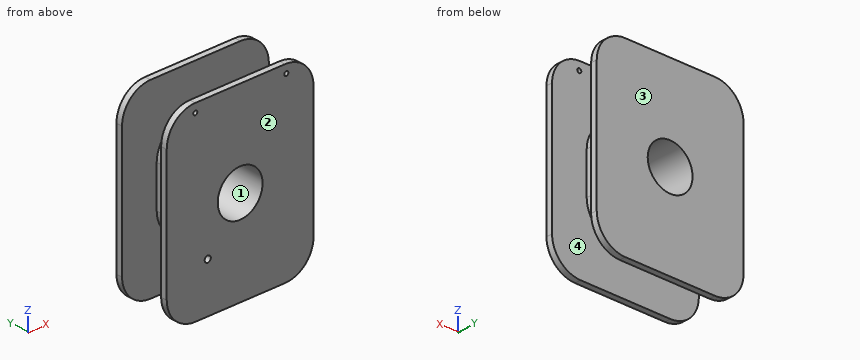
from build123d import *

# Parameters (mm, degrees)
F0_W      = 36
F0_H      = 45
F0_R      = 5.5
F1_DEPTH  = 1.5
F2_W      = 19
F2_H      = 24
F2_R      = 5.5
F3_DEPTH  = 12
F4_W      = 36
F4_H      = 45
F4_W_2    = 19
F4_H_2    = 24
F4_R      = 5.5
F5_DEPTH  = 1.5
F6_R      = 7
F7_R      = 0.75
F8_DEPTH  = 2.5
F9_R      = 0.5
F10_DEPTH = 2.5


# Not quite as in the source:
# - a feature names something its author has since deleted; it is built from what else it names


with BuildPart() as f1:
    # F0 (on Front) → F1 (new body)
    with BuildSketch(Plane.XZ):
        Rectangle(F0_W, F0_H)
        Circle(F0_R, mode=Mode.SUBTRACT)
    extrude(amount=F1_DEPTH)

    # F2 (on face) → F3 (join)
    with BuildSketch(Plane.XZ.offset(1.5)):
        Rectangle(F2_W, F2_H)
        Circle(F2_R, mode=Mode.SUBTRACT)
    extrude(amount=F3_DEPTH)

    # F4 (on face) → F5 (join)
    with BuildSketch(Plane.XZ.offset(13.5)):
        Rectangle(F4_W, F4_H)
        Rectangle(F4_W_2, F4_H_2, mode=Mode.SUBTRACT)
        Rectangle(F4_W_2, F4_H_2)
        Circle(F4_R, mode=Mode.SUBTRACT)
    extrude(amount=-F5_DEPTH)

    # F6
    f6_edges = [f1.edges().sort_by_distance(p)[0] for p in [
        (9.5, -6.75, 12),
        (9.5, -6.75, -12),
        (18, -0.75, 22.5),
        (18, -12.75, 22.5),
        (18, -12.75, -22.5),
        (18, -0.75, -22.5),
        (-18, -0.75, -22.5),
        (-18, -12.75, -22.5),
        (-9.5, -6.75, -12),
        (-9.5, -6.75, 12),
        (-18, -0.75, 22.5),
        (-18, -12.75, 22.5),
    ]]
    fillet(f6_edges, radius=F6_R)

    # F7 (on face) → F8 (cut)
    with BuildSketch(Plane.XZ.offset(13.5)):
        with Locations((-7.9445969313, -10.7102040201)):
            Circle(F7_R)
    extrude(amount=-F8_DEPTH, mode=Mode.SUBTRACT)

    # F9 (on face) → F10 (cut)
    with BuildSketch(Plane.XZ.offset(13.5)):
        with Locations((-11, 20.4497474683)):
            Circle(F9_R)
        with Locations((11.3213816658, 20.4497474683)):
            Circle(F9_R)
    extrude(amount=-F10_DEPTH, mode=Mode.SUBTRACT)


solid = f1.part
Can you work these out from the model? Positions are in its coordinate system, mm. Face numbers are marked on the shaded views. A direction names the side the tool comes from. Coordinates: 2 decimals unless noted, no trailing zeros. Write each loop counter-clockwise with the first axis right and the second up, starting at its lowest first coordinate (ties: lowest second). Pieces come first, ordered by that corner, then holes.
Q1. For P1, Ø0.9, axis at x = -7.94, z = -10.71, coming from the +Y side; P2, Ø5.5, axis at x = 1, y = -5, coming from the +Z side; P3, Ø2, axis at x = 3.5, y = -8.5, coming from the -Z side; P4, Ø3, axis at y = -7.5, z = 0, coming from the -X side, each with a flat end and sliding along its axis, tell me the tip position at first contact or that it passes through.
Results found:
P1: stops at y = 0
P2: stops at z = 12
P3: stops at z = -12
P4: stops at x = -9.5
Q2. Imagine slicing it at D-D, the plane z = 13. List the corners of the cut face in (x, y) for me, plus the area to 3 significant figures.
Results found:
outline: (-18, -13.5) - (18, -13.5) - (18, -12) - (-18, -12) - close; (-18, -1.5) - (18, -1.5) - (18, 0) - (-18, 0) - close
area: 108 mm2
Q3. Imagine slicing it at C-C, the plane x = 0. List the corners of the cut face in (y, z) for me.
Results found:
outline: (-13.5, -22.5) - (-12, -22.5) - (-12, -12) - (-1.5, -12) - (-1.5, -22.5) - (0, -22.5) - (0, -5.5) - (-13.5, -5.5) - close; (-13.5, 5.5) - (0, 5.5) - (0, 22.5) - (-1.5, 22.5) - (-1.5, 12) - (-12, 12) - (-12, 22.5) - (-13.5, 22.5) - close
Q4. Which directions (+Z, -Z, +X, -X, +Y, -Y) give clear straight access to the entire face, cutting with the end or side of a thin tool? Please do the marked faces 3 and 4.
Results found:
face 3: +Z, -Z, +X, -X, +Y
face 4: none
Q5. Imagine slicing it at B-B, the plane y = -7. List the corners of the cut face in (x, z) for me, plus the area to 3 significant figures.
Results found:
outline: (-9.5, -5) arc R7 ccw to (-2.5, -12) - (2.5, -12) arc R7 ccw to (9.5, -5) - (9.5, 5) arc R7 ccw to (2.5, 12) - (-2.5, 12) arc R7 ccw to (-9.5, 5) - close; hole circle Ø11 at (0, 0)
area: 319 mm2
Q6. Please list where these lines run through material, in increasing order: L1, parallel to Y at x = 15, z = 20.5; L2, parallel to Z at x = -11, y = -13.1; L3, parallel to Z at x = 0, y = -4.25.
Results found:
L1: y = -13.5 to -12, -1.5 to 0
L2: z = -22.5 to 19.95, 20.95 to 22.5
L3: z = -12 to -5.5, 5.5 to 12
Q7. If we mould it in two halves opening along X, with no side actions, what happens to the marked faces 1 and 2? For each: +X half, -X half, draft (parallel to the pull), parting line (faces both ways), or undercut.
Results found:
face 1: undercut
face 2: draft
Q8. Imagine slicing it at A-A, the plane z = 0. List the corners of the cut face in (x, y) for me.
Results found:
outline: (-18, -13.5) - (-5.5, -13.5) - (-5.5, 0) - (-18, 0) - (-18, -1.5) - (-9.5, -1.5) - (-9.5, -12) - (-18, -12) - close; (5.5, -13.5) - (18, -13.5) - (18, -12) - (9.5, -12) - (9.5, -1.5) - (18, -1.5) - (18, 0) - (5.5, 0) - close
